Check sheet for the drawn part. Datum: minimum x, y, z corner. Units: mm. A direction names the side the tool comes from. Round coordinates to 2 decimals unless told otherwise and drop trailing zeros. Write each loop counter-clockwise with the first axis right and the second up, starting at its lowest first coordinate (ties: lowest second). Pieces come first, ordered by that corner, then holes. Notation, with made-up numbers: (44.5, -14) - (51.5, -14) arc R23 cw to (51.5, 3) - close; hole circle Ø3 at (77, 0). An arc over 180 degrees is marked (long way). Answer as a JSON object with one key per item and string values.
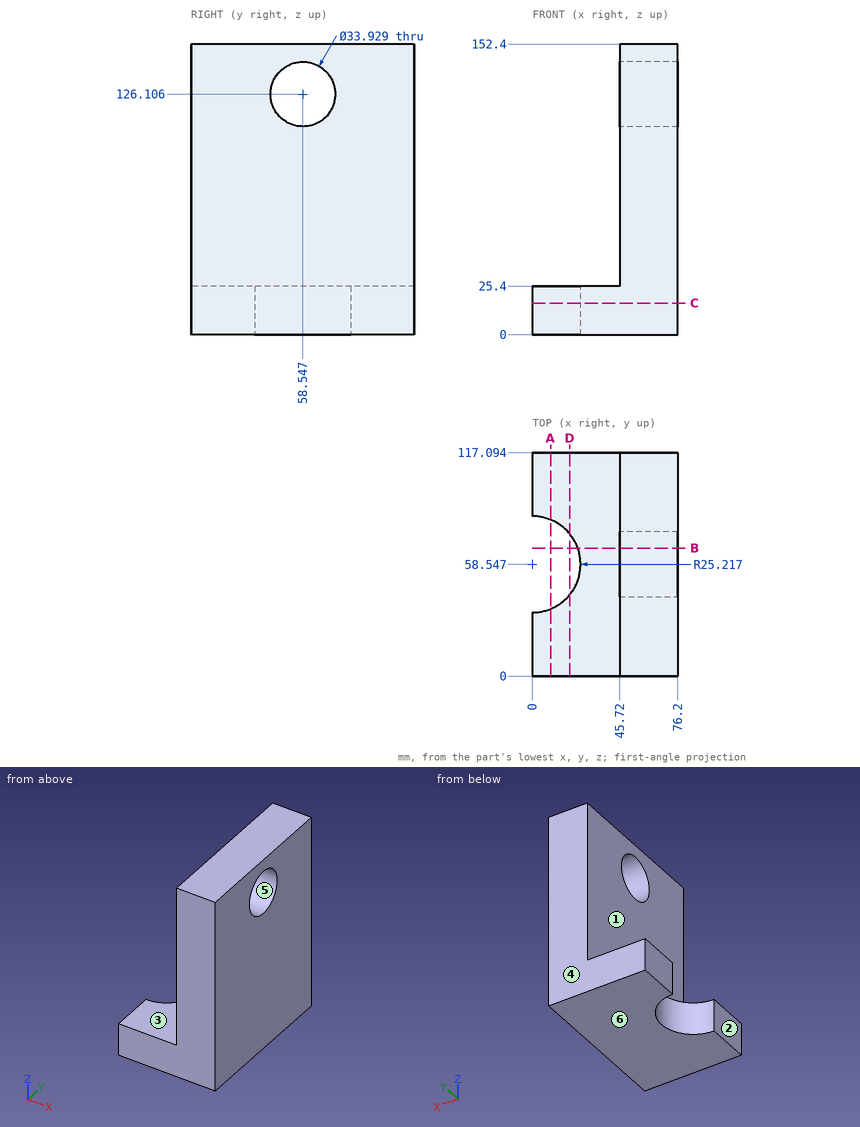
Q1. Set-up check for the marked faces 1 and 2: record each of +Z, -Z, +X, -X, +Y, -Y from which the full face is reachable in a straight line by a thin tool's end or side.
Geometry check:
{"face 1": "+Z, -X, +Y, -Y", "face 2": "+Z, -Z, -X, +Y, -Y"}
Q2. Gauge pin test, flat end, axial feed: P1, Ø2, axis at y = 83.5, z = 115, coming from the -X side. Record the tip position at first contact, or that the pin passes through.
Geometry check:
{"P1": "stops at x = 45.72"}
Q3. Section check A-A, the plane x = 9.5. Record the cut outline in (y, z).
Geometry check:
{"outline": "(0, 0) - (35.19, 0) - (35.19, 25.4) - (0, 25.4) - close; (81.91, 0) - (117.09, 0) - (117.09, 25.4) - (81.91, 25.4) - close"}
Q4. Release check for a two-part mould opening along Z. For the marked faces 3, 4, 5 and 6 record: released by +Z, released by -Z, zero draft, split by the parting line, or undercut.
Geometry check:
{"face 3": "released by +Z", "face 4": "zero draft", "face 5": "undercut", "face 6": "released by -Z"}
Q5. Section check D-D, the plane x = 19.5. Record the cut outline in (y, z).
Geometry check:
{"outline": "(0, 0) - (42.56, 0) - (42.56, 25.4) - (0, 25.4) - close; (74.54, 0) - (117.09, 0) - (117.09, 25.4) - (74.54, 25.4) - close"}
Q6. Material ranges on line 1 along X through (y, z) = (56.5, 74.5); line 2 along Z through (x, y) = (72, 57); line 3 along Z through (x, y) = (45.5, 16), recorded low to high. Write a range as [from, to].
Geometry check:
{"line 1": "x = [45.72, 76.2]", "line 2": "z = [0, 109.21], [143, 152.4]", "line 3": "z = [0, 25.4]"}
Q7. Section check B-B, the plane y = 67. Record the cut outline in (x, z), then the cut area to 3 significant figures.
Geometry check:
{"outline": "(23.76, 0) - (76.2, 0) - (76.2, 111.4) - (45.72, 111.4) - (45.72, 25.4) - (23.76, 25.4) - close; (45.72, 140.81) - (76.2, 140.81) - (76.2, 152.4) - (45.72, 152.4) - close", "area": "4,310 mm2"}
Q8. Section check C-C, the plane z = 16.5. Record the cut outline in (x, y) (1 decimal).
Geometry check:
{"outline": "(0, 0) - (76.2, 0) - (76.2, 117.1) - (0, 117.1) - (0, 83.8) arc R25.2 cw to (0, 33.3) - close"}
